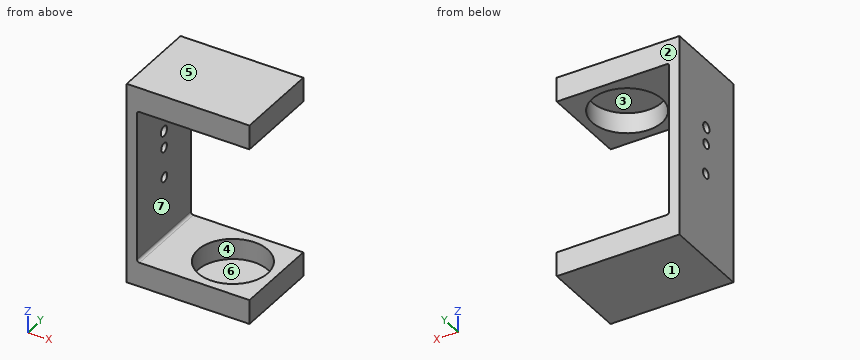
from build123d import *

# Parameters (mm, degrees)
SKETCH1_W           = 65
SKETCH1_H           = 34
SKETCH1_R           = 1.792638337
BOSS_EXTRUDE1_DEPTH = 4
SKETCH3_W           = 48
SKETCH3_H           = 34
BOSS_EXTRUDE2_DEPTH = 9.5
FILLET4_R           = 1
FILLET5_R           = 1
SKETCH5_R           = 13.65
CUT_EXTRUDE1_DEPTH  = 8
SKETCH6_R           = 1.817001486
SKETCH6_R_2         = 1.988961177
CUT_EXTRUDE2_DEPTH  = 10


with BuildPart() as part:
    # Sketch1 → Boss-Extrude1 (new body)
    with BuildSketch(Plane(origin=(0, 0, 0), x_dir=(0, 0, -1), z_dir=(1, 0, 0))):
        Rectangle(SKETCH1_W, SKETCH1_H)
        with Locations((-8.422145585, 0.13559033)):
            Circle(SKETCH1_R, mode=Mode.SUBTRACT)
    extrude(amount=-BOSS_EXTRUDE1_DEPTH)

    # Sketch3 → Boss-Extrude2 (add)
    with BuildSketch(Plane.XY.offset(32.5)):
        with Locations((20, 0)):
            Rectangle(SKETCH3_W, SKETCH3_H)
    boss_extrude2 = extrude(amount=BOSS_EXTRUDE2_DEPTH)

    # Mirror1: Boss-Extrude2 across plane
    add(boss_extrude2.mirror(Plane(origin=(0, 0, 2.5), x_dir=(1, 0, 0), z_dir=(0, 0, -1))))

    # Fillet4
    fillet4_edges = [part.edges().sort_by_distance(p)[0] for p in [
        (0, 0, 32.5),
    ]]
    fillet(fillet4_edges, radius=FILLET4_R)

    # Fillet5
    fillet5_edges = [part.edges().sort_by_distance(p)[0] for p in [
        (0, 0, -27.5),
    ]]
    fillet(fillet5_edges, radius=FILLET5_R)

    # Sketch5 → Cut-Extrude1 (cut)
    with BuildSketch(Plane(origin=(0, 0, 32.5), x_dir=(-1, 0, 0), z_dir=(0, 0, -1))):
        with Locations((-27, 0)):
            Circle(SKETCH5_R)
    cut_extrude1 = extrude(amount=-CUT_EXTRUDE1_DEPTH, mode=Mode.SUBTRACT)

    # Mirror2: Cut-Extrude1 across plane
    add(cut_extrude1.mirror(Plane(origin=(0, 0, 2.5), x_dir=(1, 0, 0), z_dir=(0, 0, -1))), mode=Mode.SUBTRACT)

    # Sketch6 → Cut-Extrude2 (cut)
    with BuildSketch(Plane.ZY.offset(4)):
        with Locations((-3.477810301, 0.314468999)):
            Circle(SKETCH6_R)
        with Locations((15.022387571, 0.02925164)):
            Circle(SKETCH6_R_2)
    extrude(amount=-CUT_EXTRUDE2_DEPTH, mode=Mode.SUBTRACT)


solid = part.part
Source: CAD feature listing. Evaluate the final solid. Frame: model axes, mm. Face numbers are marked on the shaded views. A direction names the side the tool comes from. Coordinates: 2 decimals unless noted, no trailing zeros. Order: outer loops, then holes, each group sorted by start corner. A loop starts at its lowest first (then second) coordinate and runs counter-clockwise, first axis right, second up. Notation, with made-up numbers: M -23.5,8 L 0.5,8 A10 cw 0.5,19 Z; hole C -36,44 d4. An arc over 180 degrees is marked long. Write each question's results on one line, items separated by ' | '. Start each with the question number.
Item 1: First-contact query: pin 1 Ø6 at (y, z) = (-9.5, 0.5) entering from +X. Flat tip, straight axial feed; report the tip coordinate or a pass-through.
Item 2: Set-up query: the marked faces 5, 6 and 7. Return all of +Z, -Z, +X, -X, +Y, -Y with unobstructed straight access to the full face (end or side cutting, diameter ignored); none if empty.
Item 3: Cut plane D-D (x = 27). Return loops of the section in (y, z).
Item 4: Cut plane B-B (z = 37). Return loops of the section in (x, y), and give its area (3 significant figures).
Item 5: Cut plane C-C (y = 11). Return loops of the section in (x, z), and give its area (3 significant figures).
Item 6: Draft query along Y for the marked faces 1, 2, 3 and 4. Return one class per face: pulls with the +Y half, pulls with the -Y half, needs draft (parallel to the pull), parting line crosses it, or undercut.
Item 7: Cut plane A-A (x = 4.5). Return loops of the section in (y, z).
Item 8: Line query: probe 1 along Z at (x, y) = (34, -2.5); probe 2 along Y at (x, z) = (27, 37); probe 3 along Z at (x, y) = (35, -15). Output: solid intervals per line, ascending.
Checked values:
1) pin 1: stops at x = 0
2) face 5: +Z, +X, -X, +Y, -Y | face 6: none | face 7: +X, +Y, -Y
3) outline: M -17,-37 L 17,-37 L 17,-27.5 L 13.65,-27.5 L 13.65,-35.5 L -13.65,-35.5 L -13.65,-27.5 L -17,-27.5 Z; M -17,32.5 L -13.65,32.5 L -13.65,40.5 L 13.65,40.5 L 13.65,32.5 L 17,32.5 L 17,42 L -17,42 Z
4) outline: M -4,-17 L 44,-17 L 44,17 L -4,17 Z; hole C 27,0 d27.3 | area: 1,050 mm2
5) outline: M -4,-37 L 44,-37 L 44,-27.5 L 35.08,-27.5 L 35.08,-35.5 L 18.92,-35.5 L 18.92,-27.5 L 1,-27.5 A1 cw 0,-26.5 L 0,31.5 A1 cw 1,32.5 L 18.92,32.5 L 18.92,40.5 L 35.08,40.5 L 35.08,32.5 L 44,32.5 L 44,42 L -4,42 Z | area: 894 mm2
6) face 1: needs draft | face 2: pulls with the +Y half | face 3: undercut | face 4: undercut
7) outline: M -17,-37 L 17,-37 L 17,-27.5 L -17,-27.5 Z; M -17,32.5 L 17,32.5 L 17,42 L -17,42 Z
8) probe 1: z = -37 to -35.5, 40.5 to 42 | probe 2: y = -17 to -13.65, 13.65 to 17 | probe 3: z = -37 to -27.5, 32.5 to 42
